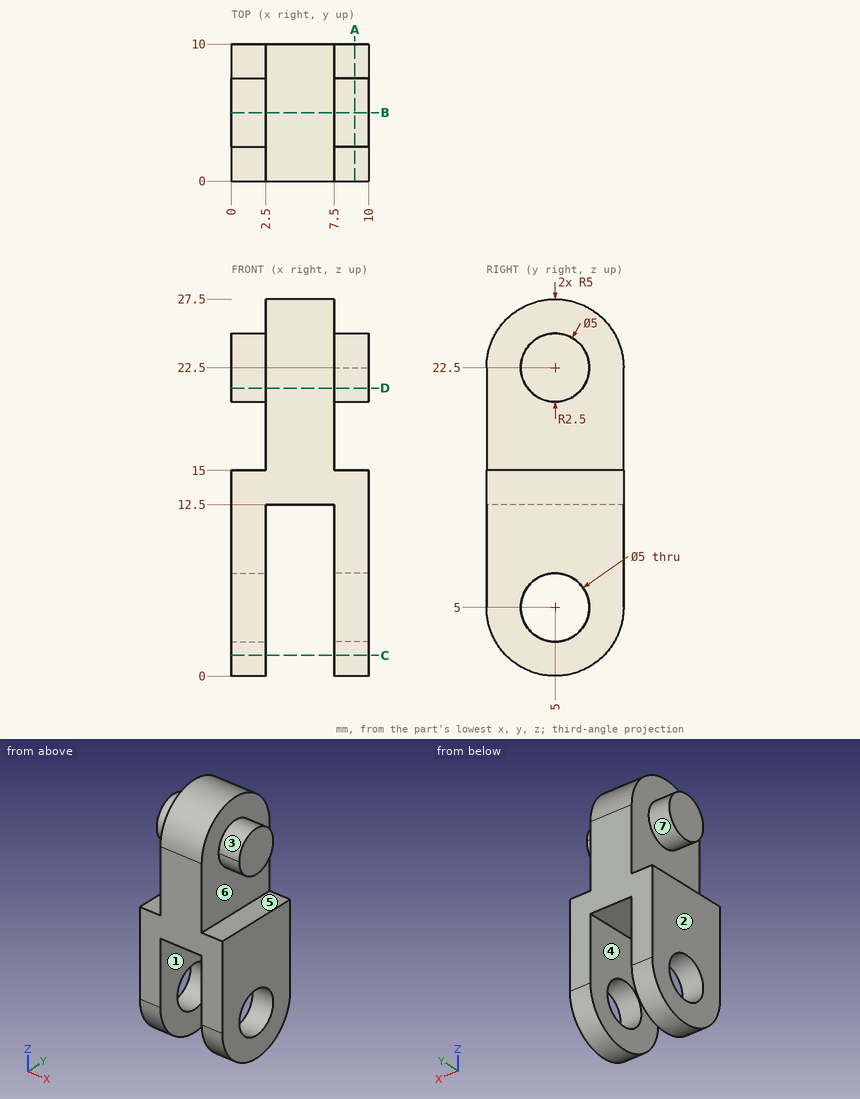
Job drawing, mm, ordinate dimensions from the low corner. One solid piece. A direction names the side the tool comes from. Give positions to 0.01 mm unless a question says otherwise; leave off trailing zeros. Write each loop counter-clockwise with the first axis right and the second up, starting at its lowest first coordinate (ties: lowest second). Pieces come first, ordered by that corner, then holes. Notation, with made-up numbers: (33.5, -7) - (42.5, -7) arc R32 cw to (42.5, 28) - close; hole circle Ø2 at (70, 16.25). An arc over 180 degrees is marked (long way). Answer as CSV lines item,"result".
1. Band-saw the part on B-B (y = 5). Write the cut outline in (x, z).
Responses:
outline,"(0, 0) - (2.5, 0) - (2.5, 2.5) - (0, 2.5) - close; (0, 7.5) - (2.5, 7.5) - (2.5, 12.5) - (7.5, 12.5) - (7.5, 7.5) - (10, 7.5) - (10, 15) - (7.5, 15) - (7.5, 20) - (10, 20) - (10, 25) - (7.5, 25) - (7.5, 27.5) - (2.5, 27.5) - (2.5, 25) - (0, 25) - (0, 20) - (2.5, 20) - (2.5, 15) - (0, 15) - close; (7.5, 0) - (10, 0) - (10, 2.5) - (7.5, 2.5) - close"
2. 3-axis set-ups, long thin cutter, end or side, ignore diameter. For the marked faces 4, 5, 6 and 7: which of +Z, -Z, +X, -X, +Y, -Y reach the whole face in a straight line?
Responses:
face 4,"-Z, +Y, -Y"
face 5,"+X, +Y, -Y"
face 6,"+X"
face 7,"-X"
3. Pin check, flat tips, straight feed: pin 1 (2 mm diameter, centred on x = 1, y = 4.5, fed in from +Z); pin 2 (0.8 mm diameter, centred on x = 9, y = 7.5, fed in from +Z); pin 3 (4 mm diameter, centred on x = 1, y = 5.5, fed in from -Z); pin 4 (3 mm diameter, centred on y = 5, z = 5, fed in from +X). Stop position of each tip, or through.
Responses:
pin 1,"stops at z = 25"
pin 2,"stops at z = 23.86"
pin 3,"stops at z = 0"
pin 4,"passes through"
4. Band-saw the part on D-D (z = 21). Write the cut outline in (x, y), and give its area (3 significant figures).
Responses:
outline,"(0, 3) - (2.5, 3) - (2.5, 0) - (7.5, 0) - (7.5, 3) - (10, 3) - (10, 7) - (7.5, 7) - (7.5, 10) - (2.5, 10) - (2.5, 7) - (0, 7) - close"
area,"70.0 mm2"
5. Drill centre lines: L1, parallel to Z at x = 8.5, y = 5; L2, parallel to Y at x = 1.4, z = 5; L3, parallel to Z at x = 0.5, y = 6.5. Where is each one in solid material? Low to high. Write a range as [from, to].
Responses:
L1,"z = [0, 2.5], [7.5, 15], [20, 25]"
L2,"y = [0, 2.5], [7.5, 10]"
L3,"z = [0.23, 3], [7, 15], [20.5, 24.5]"
6. Band-saw the part on C-C (z = 1.5). Write the cut outline in (x, y), and give its area (3 significant figures).
Responses:
outline,"(0, 1.43) - (2.5, 1.43) - (2.5, 8.57) - (0, 8.57) - close; (7.5, 1.43) - (10, 1.43) - (10, 8.57) - (7.5, 8.57) - close"
area,"35.7 mm2"
7. Two-plate mould, pull along X, no slides. Class the marked faces 1, 2 and 3: +X half, -X half, draft (parallel to the pull), parting line (faces both ways), or undercut.
Responses:
face 1,"undercut"
face 2,"-X half"
face 3,"draft"
8. Band-saw the part on A-A (x = 9). Count the separate pieces of the cut face and the enclosed holes in it, and give its area (3 significant figures).
Responses:
separate pieces,"2"
enclosed holes,"1"
area,"139 mm2"
